Here's the drawing with two shaded views (mm, measured from the low corner). I have some questions. A direction names the side the tool comes from. Give positions to 0.01 mm unless a question says otherwise; leave off trailing zeros. Loops run counter-clockwise (first coordinate to the right, second up) from the corner with the lowest first, then second, coordinate; pieces in that order, holes last. Notation, with made-up numbers: M -4.5,-5.75 L 21.5,-5.75 A27 ccw 21.5,30.25 Z; hole C 85,25 d5. An arc over 180 degrees is marked long. Put each result on its own line as item: value. Start each with the question number.
1) Imagine slicing it at C-C (z = 4.5). Write out the boundary of the cut face in (x, y).
2) Imagine slicing it at A-A (x = 2.5). Write out the boundary of the cut face in (y, z), then the cut area to 3 significant figures.
3) Imagine slicing it at B-B (y = 3.25). Write out the boundary of the cut face in (x, z), then the cut area to 3 significant figures.
4) For P1, Ø0.8, axis at y = 3.5, z = 3, coming from the +X side, with a flat end and sliding along its axis, tell me the tip position at first contact or that it passes through.
5) Imagine slicing it at D-D (y = 9). Write out the boundary of the cut face in (x, z), then the cut area to 3 significant figures.
6) For the marked faces 1, 2 and 3, which set-ups out of +Z, -Z, +X, -X, +Y, -Y let a thin tool reach every point of the face, with its end or its side?
7) If we mould it in two halves opening along Z, with no side actions, what happens to the marked faces 4, 5 and 6? For each: +Z half, -Z half, draft (parallel to the pull), parting line (faces both ways), or undercut.
8) Please list where these lines run through material, in increasing order: line 1 along Z through (x, y) = (4, 9); line 2 along Y through (x, z) = (1.75, 4.5); line 3 along Y through (x, z) = (1, 4.45). Write a range as from..to.
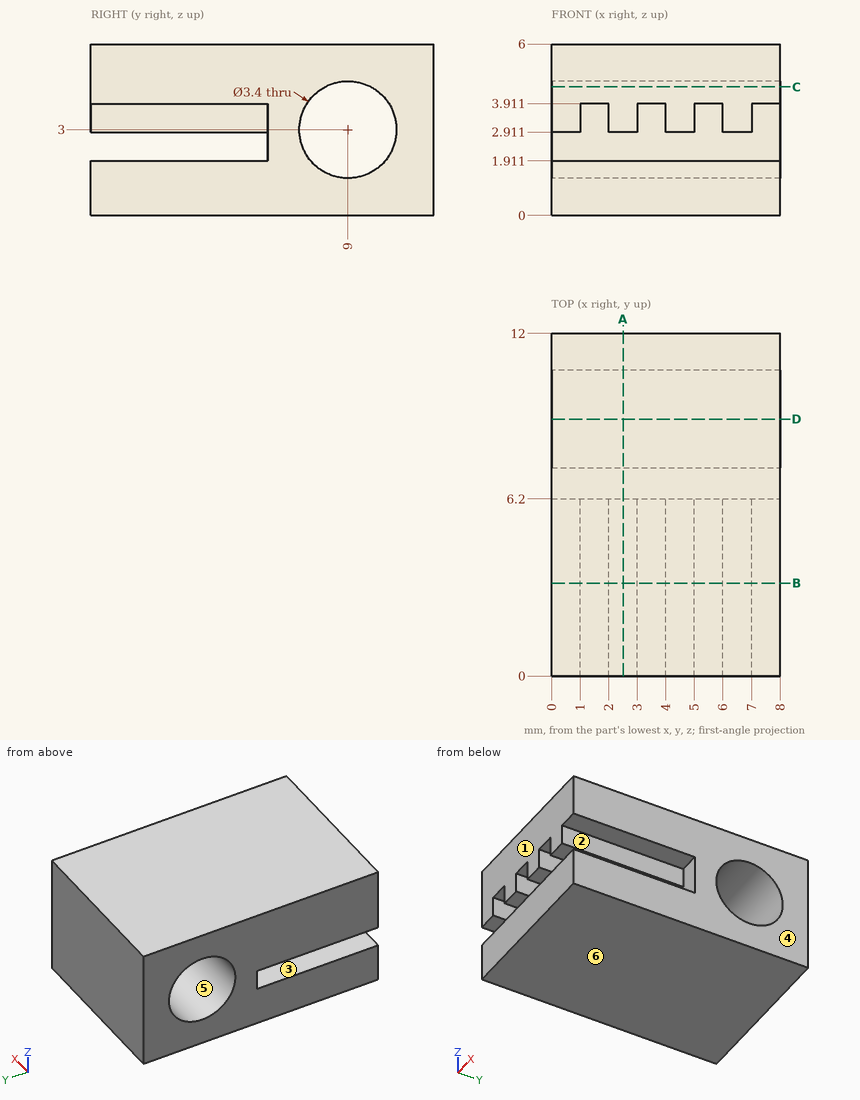
Recorded:
1. outline: M 0,0 L 8,0 L 8,8.2 L 0,8.2 Z; M 0,9.8 L 8,9.8 L 8,12 L 0,12 Z
2. outline: M 0,0 L 12,0 L 12,6 L 0,6 L 0,2.91 L 6.2,2.91 L 6.2,1.91 L 0,1.91 Z; hole C 9,3 d3.4
2. area: 56.7 mm²
3. outline: M 0,0 L 8,0 L 8,1.91 L 0,1.91 Z; M 0,2.91 L 1,2.91 L 1,3.91 L 2,3.91 L 2,2.91 L 3,2.91 L 3,3.91 L 4,3.91 L 4,2.91 L 5,2.91 L 5,3.91 L 6,3.91 L 6,2.91 L 7,2.91 L 7,3.91 L 8,3.91 L 8,6 L 0,6 Z
3. area: 36.0 mm²
4. P1: x = 7
5. outline: M 0,0 L 8,0 L 8,1.3 L 0,1.3 Z; M 0,4.7 L 8,4.7 L 8,6 L 0,6 Z
5. area: 20.8 mm²
6. face 1: +Z, -Z, +X, -X, -Y
6. face 2: +X, -Y
6. face 3: +X, -X, -Y
7. face 4: draft
7. face 5: undercut
7. face 6: -Z half
8. line 1: 0..1.3, 4.7..6
8. line 2: 0..8.2, 9.8..12
8. line 3: 0..8.11, 9.89..12
